The model under review builds one solid part; all positions refer to its coordinate system, in mm. A direction names the side the tool comes from. Round coordinates to 2 decimals unless told otherwise and drop trailing zeros. Order: outer loops, then holes, each group sorted by start corner. A loop starts at its lowest first (then second) coordinate and runs counter-clockwise, first axis right, second up. Notation, with made-up numbers: M -4,-26.5 L 28,-26.5 A11 ccw 28,-17.5 Z; hole C -21.5,84.25 d7. An arc over 180 degrees is marked long. Answer as a JSON object with one key per item and string values. Group by question number.
1) Consider section D-D, the plane z = 7.5. Write out the cut boundary in (x, y).
2) To check wall thickness, follow line 1 (X direction, y = -5, z = 3.5); line 2 (Y direction, x = -0.5, z = 15); line 3 (Y direction, x = 1, z = 8). State the ranges of each line that lie inside material, in increasing order.
3) Consider section B-B, the plane x = -4.5. Write out the cut boundary in (y, z).
4) Insertion check: pin 1 Ø1.6 at (y, z) = (-2.97, 14.8) entering from -X; pin 2 Ø5 at (x, y) = (-1.5, -2) entering from -Z. Each pin has a flat end and moves straight along its axis. Give the tip position at first contact, or say it passes through.
5) The part is to be moulded in two halves that separate along X. For faces 1 (the cylindrical face through (0.165, 6.993, 8.964)), 2 (the flat face through (-7.01, 0, 22)), 3 (the cylindrical face through (-6.271, -2.667, 15.754)), 4 (the flat face through (0, -5.767, 22)), say which applies: +X half, -X half, draft (parallel to the pull), parting line (faces both ways), or undercut.
6) Consider section C-C, the plane z = 25.6. Write out the cut boundary in (x, y), then the cut area to 3 significant figures.
7) For faces 5 (the cylindrical face through (0.165, -6.528, 36.036)), 6 (the cylindrical face through (-6.27, -2.92, 24.6)), 7 (the flat face through (0, 6.233, 22)), list the 3-axis set-ups (+Z, -Z, +X, -X, +Y, -Y) from which the entire face can be reached by the end or side of a thin tool; tool diameter is ignored.
8) Consider section A-A, the plane y = 5.75. Write out the cut boundary in (x, z).
```python
from build123d import *

# Parameters (mm, degrees)
SKETCH_1_W          = 15
SKETCH_1_H          = 15
SKETCH_1_W_2        = 12
SKETCH_1_H_2        = 12
EXTRUDE_2_DEPTH     = 45
SKETCH_2_R          = 1.5
CUT_EXTRUDE_1_DEPTH = 10
SKETCH_3_R          = 1.5
CUT_EXTRUDE_2_DEPTH = 10
SKETCH_7_R          = 1
CUT_EXTRUDE_5_DEPTH = 10


with BuildPart() as part:
    # ｽｹｯﾁ1 → ﾎﾞｽ - 押し出し2 (new body)
    with BuildSketch(Plane.XY):
        with Locations((0.489915859, 0.232626086)):
            Rectangle(SKETCH_1_W, SKETCH_1_H)
        with Locations((0.489915859, 0.232626086)):
            Rectangle(SKETCH_1_W_2, SKETCH_1_H_2, mode=Mode.SUBTRACT)
    extrude(amount=EXTRUDE_2_DEPTH)

    # ｽｹｯﾁ2 → ｶｯﾄ - 押し出し1 (cut)
    with BuildSketch(Plane(origin=(0, 7.732626086, 0), x_dir=(1, 0, 0), z_dir=(0, 1, 0))):
        with Locations((0.489915859, -7.5)):
            Circle(SKETCH_2_R)
    extrude(amount=-CUT_EXTRUDE_1_DEPTH, mode=Mode.SUBTRACT)

    # ｽｹｯﾁ3 → ｶｯﾄ - 押し出し2 (cut)
    with BuildSketch(Plane.XZ.offset(7.267373914)):
        with Locations((0.489915859, 37.5)):
            Circle(SKETCH_3_R)
    extrude(amount=-CUT_EXTRUDE_2_DEPTH, mode=Mode.SUBTRACT)

    # ｽｹｯﾁ7 → ｶｯﾄ - 押し出し5 (cut)
    with BuildSketch(Plane.ZY.offset(7.010084141)):
        with Locations((25.6, -2.967373914)):
            Circle(SKETCH_7_R)
        with Locations((14.8, -2.967373914)):
            Circle(SKETCH_7_R)
    extrude(amount=-CUT_EXTRUDE_5_DEPTH, mode=Mode.SUBTRACT)


solid = part.part
```
Results list:
{
 "1": {"outline": "M -7.01,-7.27 L 7.99,-7.27 L 7.99,7.73 L 1.99,7.73 L 1.99,6.23 L 6.49,6.23 L 6.49,-5.77 L -5.51,-5.77 L -5.51,6.23 L -1.01,6.23 L -1.01,7.73 L -7.01,7.73 Z"},
 "2": {"line 1": "-7.01 to -5.51, 6.49 to 7.99", "line 2": "-7.27 to -5.77, 6.23 to 7.73", "line 3": "-7.27 to -5.77"},
 "3": {"outline": "M -7.27,0 L -5.77,0 L -5.77,45 L -7.27,45 Z; M 6.23,0 L 7.73,0 L 7.73,45 L 6.23,45 Z"},
 "4": {"pin 1": "x = 6.49", "pin 2": "through"},
 "5": {"face 1": "undercut", "face 2": "-X half", "face 3": "draft", "face 4": "undercut"},
 "6": {"outline": "M -7.01,-7.27 L 7.99,-7.27 L 7.99,7.73 L -7.01,7.73 L -7.01,-1.97 L -5.51,-1.97 L -5.51,6.23 L 6.49,6.23 L 6.49,-5.77 L -5.51,-5.77 L -5.51,-3.97 L -7.01,-3.97 Z", "area": "78.0 mm^2"},
 "7": {"face 5": "-Y", "face 6": "-X", "face 7": "+Z, -Z"},
 "8": {"outline": "M -7.01,0 L -5.51,0 L -5.51,45 L -7.01,45 Z; M 6.49,0 L 7.99,0 L 7.99,45 L 6.49,45 Z"}
}
